The model under review builds one solid part; all positions refer to its coordinate system, in mm. A direction names the side the tool comes from. Give positions to 0.01 mm unless a question says otherwise; leave off trailing zeros. Loops run counter-clockwise (first coordinate to the right, second up) from the corner with the lowest first, then second, coordinate; pieces in that order, holes last. Notation, with made-up numbers: M 3.5,-7.5 L 14.5,-7.5 A32 cw 14.5,25.5 Z; hole C 23.25,81 d2. An arc over 180 degrees is marked long. One line per item, written item: value. Start each with the question number.
Q1. For pin 1 (12 mm diameter, centred on x = 28, y = -12, fed in from +Z); pin 2 (3 mm diameter, centred on x = -40, z = -1.5, fed in from -Y); pin 3 (5.5 mm diameter, centred on x = -21.2, y = 29, fed in from -Z); pin 4 (0.9 mm diameter, centred on x = -2, z = 1, fed in from +Y), all flat-tipped, find the tip position at first contact; note any pin that passes through.
Q2. To check wall thickness, follow line 1 along Y through (x, z) = (-21.2, -3.2); line 2 along Y through (x, z) = (42.5, -1.8) (3 decimals); line 3 along Y through (x, z) = (0, -3.4). State the ranges of each line that lie inside material, in increasing order. Write a range as from..to.
Q3. We need section D-D on x = 21.2. Write out the cut boundary in (y, z).
Q4. We need section C-C on y = 15. Write out the cut boundary in (x, z) (3 decimals).
Q5. Mouldability with a two-part tool opening along X and no side actions: class faces 4 (the face through (48, 32.9, -3)), 5 (the face through (21, -32.557, -1)), 6 (the face through (0, 15, 3)) as released by +X, released by -X, zero draft, split by the parting line, or undercut.
Q6. For faces 1 (the face through (-24.167, -27.283, -1.232)), 2 (the face through (-22.7, -27.6, -4.2)), 3 (the face through (30, 15, 1)), list the 3-axis set-ups (+Z, -Z, +X, -X, +Y, -Y) from which the entire face can be reached by the end or side of a thin tool; tool diameter is ignored.
Q7. We need section B-B on x = 0. Write out the cut boundary in (y, z), plus the area to 4 significant figures.
Q8. We need section A-A on y = -11. Write out the cut boundary in (x, z).
```python
from build123d import *

# Parameters (mm, degrees)
F0_R      = 2.05
F1_DEPTH  = 6
F2_R      = 2.125
F2_W      = 60
F2_H      = 7.5
F3_DEPTH  = 6
F5_DEPTH  = 2.5
F6_DEPTH  = 25
F7_SIZE   = 1.9
F8_DEPTH  = 3
F9_R      = 17.5
F10_DEPTH = 25


# Not quite as in the source:
# - a feature names something its author has since deleted; it is built from what else it names


with BuildPart() as f1:
    # F0 (on Top) → F1 (new body)
    with BuildSketch(Plane.XY):
        with BuildLine():
            ThreePointArc((35, 27), (32.6568542495, 32.6568542495), (27, 35))
            Line((27, 35), (-27, 35))
            ThreePointArc((-27, 35), (-32.6568542495, 32.6568542495), (-35, 27))
            Line((-35, 27), (-35, -27))
            ThreePointArc((-35, -27), (-32.6568542495, -32.6568542495), (-27, -35))
            Line((-27, -35), (27, -35))
            ThreePointArc((27, -35), (32.6568542495, -32.6568542495), (35, -27))
            Line((35, -27), (35, 27))
        make_face()
        with Locations((-21.2, -29)):
            Circle(F0_R, mode=Mode.SUBTRACT)
        with Locations((21.2, -29)):
            Circle(F0_R, mode=Mode.SUBTRACT)
        with Locations((-21.2, 29)):
            Circle(F0_R, mode=Mode.SUBTRACT)
        with Locations((21.2, 29)):
            Circle(F0_R, mode=Mode.SUBTRACT)
        with Locations((-21.2, 29)):
            Circle(F0_R)
        with Locations((21.2, 29)):
            Circle(F0_R)
        with Locations((21.2, -29)):
            Circle(F0_R)
        with Locations((-21.2, -29)):
            Circle(F0_R)
    extrude(amount=-F1_DEPTH)

    # F2 (on Top) → F3 (join)
    with BuildSketch(Plane.XY):
        with BuildLine():
            ThreePointArc((50, 28), (47.9497474683, 32.9497474683), (43, 35))
            Line((43, 35), (-43, 35))
            ThreePointArc((-43, 35), (-47.9497474683, 32.9497474683), (-50, 28))
            Line((-50, 28), (-50, 2))
            ThreePointArc((-50, 2), (-47.9497474683, -2.9497474683), (-43, -5))
            Line((-43, -5), (43, -5))
            ThreePointArc((43, -5), (47.9497474683, -2.9497474683), (50, 2))
            Line((50, 2), (50, 28))
        make_face()
        with Locations((-42.5, 15)):
            Circle(F2_R, mode=Mode.SUBTRACT)
        with Locations((0, 15)):
            Rectangle(F2_W, F2_H, mode=Mode.SUBTRACT)
        with Locations((42.5, 15)):
            Circle(F2_R, mode=Mode.SUBTRACT)
    extrude(amount=-F3_DEPTH)

    # F4 (on Top) → F5 (cut)
    with BuildSketch(Plane.XY):
        Polygon((19.1289578016, -32.5574766695), (23.1704096859, -32.5574766695), (25.191135628, -29.0574766695), (23.1704096859, -25.5574766695), (19.1289578016, -25.5574766695), (17.1082318594, -29.0574766695), align=None)
        Polygon((-17.1082318594, -29.0574766695), (-19.1289578016, -25.5574766695), (-23.1704096859, -25.5574766695), (-25.191135628, -29.0574766695), (-23.1704096859, -32.5574766695), (-19.1289578016, -32.5574766695), align=None)
        Polygon((-23.1704096859, 25.5574766695), (-19.1289578016, 25.5574766695), (-17.1082318594, 29.0574766695), (-19.1289578016, 32.5574766695), (-23.1704096859, 32.5574766695), (-25.191135628, 29.0574766695), align=None)
        Polygon((19.1289578016, 32.5574766695), (17.1082318594, 29.0574766695), (19.1289578016, 25.5574766695), (23.1704096859, 25.5574766695), (25.191135628, 29.0574766695), (23.1704096859, 32.5574766695), align=None)
    extrude(amount=-F5_DEPTH, mode=Mode.SUBTRACT)

    # F0 (on Top) → F6 (cut)
    with BuildSketch(Plane.XY):
        with Locations((-21.2, 29)):
            Circle(F0_R)
        with Locations((21.2, 29)):
            Circle(F0_R)
        with Locations((21.2, -29)):
            Circle(F0_R)
        with Locations((-21.2, -29)):
            Circle(F0_R)
    extrude(amount=-F6_DEPTH, mode=Mode.SUBTRACT)

    # F7
    f7_edges = [f1.edges().sort_by_distance(p)[0] for p in [
        (40.375, 15, -6),
        (-44.625, 15, -6),
    ]]
    chamfer(f7_edges, length=F7_SIZE)

    # F2 (on Top) → F8 (join)
    with BuildSketch(Plane.XY):
        with Locations((0, 15)):
            Rectangle(F2_W, F2_H)
    extrude(amount=F8_DEPTH)

    # F9 (on Top) → F10 (cut)
    with BuildSketch(Plane.XY):
        with Locations((0, -11)):
            Circle(F9_R)
    extrude(amount=-F10_DEPTH, mode=Mode.SUBTRACT)


solid = f1.part
```
Solved:
1. pin 1: z = 0
1. pin 2: y = -5
1. pin 3: z = -6
1. pin 4: y = 18.75
2. line 1: -35..-31.05, -26.95..26.95, 31.05..35
2. line 2: -5..12.875, 17.125..35
2. line 3: -35..-28.5, 6.5..35
3. outline: M -35,-6 L -31.05,-6 L -31.05,-2.5 L -32.56,-2.5 L -32.56,0 L -35,0 Z; M -26.95,-6 L 26.95,-6 L 26.95,-2.5 L 25.56,-2.5 L 25.56,0 L 18.75,0 L 18.75,3 L 11.25,3 L 11.25,0 L -25.56,0 L -25.56,-2.5 L -26.95,-2.5 Z; M 31.05,-6 L 35,-6 L 35,0 L 32.56,0 L 32.56,-2.5 L 31.05,-2.5 Z
4. outline: M -50,-6 L -46.525,-6 L -44.625,-4.1 L -44.625,0 L -50,0 Z; M -40.375,-4.1 L -38.475,-6 L 38.475,-6 L 40.375,-4.1 L 40.375,0 L 30,0 L 30,3 L -30,3 L -30,0 L -40.375,0 Z; M 44.625,-4.1 L 46.525,-6 L 50,-6 L 50,0 L 44.625,0 Z
5. face 4: released by +X
5. face 5: undercut
5. face 6: zero draft
6. face 1: +Z
6. face 2: +Z, -Z
6. face 3: +Z, +X, +Y, -Y
7. outline: M -35,-6 L -28.5,-6 L -28.5,0 L -35,0 Z; M 6.5,-6 L 35,-6 L 35,0 L 18.75,0 L 18.75,3 L 11.25,3 L 11.25,0 L 6.5,0 Z
7. area: 232.5 mm2
8. outline: M -35,-6 L -17.5,-6 L -17.5,0 L -35,0 Z; M 17.5,-6 L 35,-6 L 35,0 L 17.5,0 Z
